Work out the finished part from the listing and answer in its coordinate system (mm). A direction names the side the tool comes from. Coordinates: 2 decimals unless noted, no trailing zeros. Order: outer loops, then holes, each group sorted by start corner. A loop starts at its lowest first (then second) coordinate and runs counter-clockwise, first axis right, second up. Notation, with made-up numbers: M -30,61 L 4,61 A32 cw 4,94 Z; hole C 48,-35.5 d5. An arc over 180 degrees is marked long. Answer in a Markdown table with one row per item. Add a question column.
Item 1: The mould has two halves that part along Z. Classify faces 6 (the face through (15.954, 6.261, -6.894)), 7 (the face through (3.75, 6.44, 4.63)), 8 (the face through (6.719, 6.261, -3.727)), 9 (the face through (9, 0, 0)): released by +Z, released by -Z, zero draft, split by the parting line, or undercut.
Item 2: Which of the six approach directions +Z, -Z, +X, -X, +Y, -Y give full straight-line access (tool end or side, diameter ignored) to faces 1 (the face through (5, 3.175, -29)), 2 (the face through (7, -22.225, -18)), 3 (the face through (7.732, -4.518, -9.267)), 4 (the face through (14.81, 6.44, 7.02)), 5 (the face through (5.05, -9.7, -27.45))?
Item 3: The part is cut by section A-A (y = -21). Write down the section's boundary in (x, z), then the cut area to 3 significant figures.
Item 4: Consider line 1 (Z direction, x = 12, y = 2.5); line 2 (X direction, y = 9, z = 0) (1 decimal); line 3 (Y direction, x = 4.5, z = -26.5) (3 decimals). Determine where each line is inside the solid, lowest interval first. Write a range as from..to.
Item 5: The part is cut by section B-B (z = 2). Write down the section's boundary in (x, y).
Item 6: The part is cut by section C-C (x = 13). Write down the section's boundary in (y, z) (1 decimal), then the cut area to 3 significant figures.
Item 7: Flat-ended cylindrical pins translate along their axes: pin 1 Ø12 at (x, z) = (22.5, -1) entering from +Y; pin 2 Ø6 at (x, y) = (12, 8) entering from +Z; pin 3 Ø4 at (x, z) = (3, -27.5) entering from +Y (3 decimals); pin 4 Ø3 at (x, y) = (1.5, 8.5) entering from +Z. Find the tip coordinate at first contact, or state that the pin passes through.
Item 8: The part is cut by section D-D (y = 7.5). Write down the section's boundary in (x, z) (1 decimal).
from build123d import *

# Parameters (mm, degrees)
BOSS_EXTRUDE1_DEPTH = 12.7
SKETCH2_R           = 4.445
SKETCH2_R_2         = 6.3754
CUT_EXTRUDE1_DEPTH  = 32.324143561
BOSS_EXTRUDE2_DEPTH = 38.1
SKETCH6_W           = 31.377120578
SKETCH6_H           = 3.175
BOSS_EXTRUDE5_DEPTH = 21.59
BOSS_EXTRUDE6_DEPTH = 25.4
CUT_EXTRUDE3_DEPTH  = 58.023970058


with BuildPart() as part:
    # Sketch1 → Boss-Extrude1 (new body)
    with BuildSketch(Plane(origin=(0, 0, 0), x_dir=(1, 0, 0), z_dir=(0, 1, 0))):
        with BuildLine():
            ThreePointArc((7.527044942, 1.542649246), (-7.678390875, -0.2801532), (7.619451552, -0.990015299))
            ThreePointArc((7.619451552, -0.990015299), (26.729936345, 0.975266474), (7.527044942, 1.542649246))
        make_face()
    extrude(amount=BOSS_EXTRUDE1_DEPTH)

    # Sketch2 → Cut-Extrude1 (cut, through all)
    with BuildSketch(Plane.XZ):
        with Locations(Location((0, 0, 0), (0, 0, 270))):
            Circle(SKETCH2_R)
        with Locations(Location((17.109737529, -0.624264614, 0), (0, 0, 270))):
            Circle(SKETCH2_R_2)
    extrude(amount=-CUT_EXTRUDE1_DEPTH, mode=Mode.SUBTRACT)

    # Sketch3 → Boss-Extrude2 (add)
    with BuildSketch(Plane(origin=(0, 12.7, 0), x_dir=(1, 0, 0), z_dir=(0, 1, 0))):
        Polygon((-7.5722719, 7.013696287), (23.470212778, 11.584018023), (23.943763832, 8.367570213), (-7.098720846, 3.797248478), align=None)
    extrude(amount=-BOSS_EXTRUDE2_DEPTH)

    # Sketch6 → Boss-Extrude5 (add)
    with BuildSketch(Plane(origin=(-1.171358862, 0, -7.956089665), x_dir=(-0.989335034779027, 0, 0.14565778028921603), z_dir=(-0.14565778028921603, 0, -0.989335034779027))):
        with Locations((-9.218645838, -23.8125)):
            Rectangle(SKETCH6_W, SKETCH6_H)
    extrude(amount=BOSS_EXTRUDE5_DEPTH)

    # Sketch7 → Boss-Extrude6 (add)
    with BuildSketch(Plane(origin=(0, -22.225, 0), x_dir=(1, 0, 0), z_dir=(0, 1, 0))):
        Polygon((-10.717023377, 28.373439688), (-10.249574599, 25.198439688), (20.792910079, 29.768761424), (20.325461302, 32.943761424), align=None)
    extrude(amount=BOSS_EXTRUDE6_DEPTH)

    # Sketch8 → Cut-Extrude3 (cut, through all)
    with BuildSketch(Plane(origin=(0, 12.7, 0), x_dir=(1, 0, 0), z_dir=(0, 1, 0))):
        Polygon((-2.52817795, -3.656000718), (3.474592527, -2.772225058), (4.3267986, -8.560568969), (-1.675971877, -9.444344629), align=None)
        Polygon((14.542367287, -5.211344626), (21.250041443, -4.223787434), (21.957699633, -9.030334935), (15.250025476, -10.017892127), align=None)
    extrude(amount=-CUT_EXTRUDE3_DEPTH, mode=Mode.SUBTRACT)


solid = part.part
Reply:
| question | item | result |
|---|---|---|
| 1 | face 6 | undercut |
| 1 | face 7 | released by +Z |
| 1 | face 8 | undercut |
| 1 | face 9 | zero draft |
| 2 | face 1 | -Z, +X, -X, +Y |
| 2 | face 2 | +Y |
| 2 | face 3 | -X, +Y |
| 2 | face 4 | +Y, -Y |
| 2 | face 5 | +X, +Y |
| 3 | outline | M -10.72,-28.37 L 20.33,-32.94 L 20.79,-29.77 L -10.25,-25.2 Z; M -7.57,-7.01 L 23.47,-11.58 L 23.94,-8.37 L -7.1,-3.8 Z |
| 3 | area | 203 mm2 |
| 4 | line 1 | z = -31.72..-28.47, -9.9..-4.44, 3.19..7.53 |
| 4 | line 2 | x = -7.7..-4.4, 4.4..10.8, 23.5..26.7 |
| 4 | line 3 | y = -25.4..-22.225 |
| 5 | outline | M -7.42,0 L -3.97,0 L -3.97,12.7 L -7.42,12.7 Z; M 3.97,0 L 7.42,0 L 7.42,12.7 L 3.97,12.7 Z; M 7.85,0 L 11.3,0 L 11.3,12.7 L 7.85,12.7 Z; M 22.92,0 L 26.37,0 L 26.37,12.7 L 22.92,12.7 Z |
| 6 | outline | M -25.4,-31.9 L 3.2,-31.9 L 3.2,-28.6 L -22.2,-28.6 L -22.2,-10 L 12.7,-10 L 12.7,-5.5 L 0,-5.5 L 0,-6.8 L -25.4,-6.8 Z; M 0,4.2 L 12.7,4.2 L 12.7,8.1 L 0,8.1 Z |
| 6 | area | 342 mm2 |
| 7 | pin 1 | stops at y = 12.7 |
| 7 | pin 2 | stops at z = 8.77 |
| 7 | pin 3 | stops at y = 3.175 |
| 7 | pin 4 | stops at z = -3.28 |
| 8 | outline | M -7.6,-7 L 23.5,-11.6 L 23.9,-8.4 L 23,-8.2 A9.6 ccw 21.8,7.8 L 21.3,4.2 A6.4 cw long 14.5,5.2 L 15.1,8.8 A9.6 ccw 7.6,1 A7.7 ccw 4,6.5 L 3.5,2.8 A4.4 cw long -2.5,3.7 L -2,7.4 A7.7 ccw -6.6,-3.9 L -7.1,-3.8 Z; hole M 5.2,-5.6 L 9.3,-6.2 A9.6 cw 7.5,-1.5 A7.7 cw Z |
